Work out the finished part from the listing and answer in its coordinate system (mm). Face numbers are marked on the shaded views. A direction names the side the tool comes from. Coordinates: 2 decimals unless noted, no trailing zeros. Write item = value, one per line. Start each with the question number.
Q1. This flat-tipped pin is pushed along its axis until it touches: P1, Ø2, axis at y = 19.5, z = 2, coming from the -X side. Where does it stop, or does it pass through?
Q2. A tool of negligible diameter and unlimited length cuts with its end or side. For the marked faces 1 and 2, from which of +Z, -Z, +X, -X, +Y, -Y can it reach the whole face along a straight path? Write none if from no direction.
Q3. Straight lines are drawn through the part: line 1 along X through (y, z) = (29, 3); line 2 along X through (y, z) = (-27, 3.15); line 3 along Y through (x, z) = (-23.5, 3.65). For each, find the intervals that lie inside material, in ascending order.
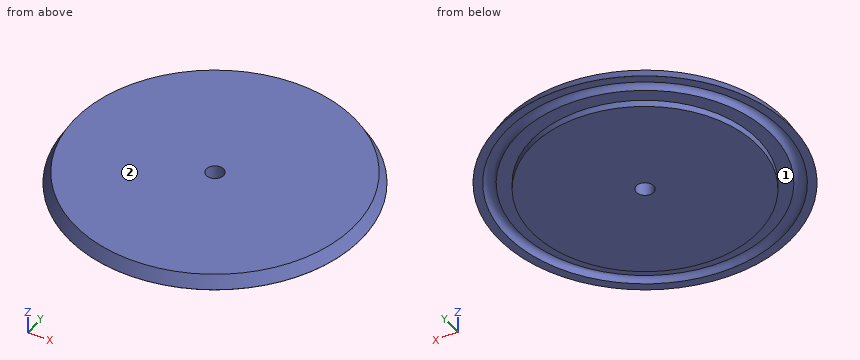
```python
from build123d import *

# Parameters (mm, degrees)
F2_R     = 2.6
F3_DEPTH = 5.501
F4_SIZE2 = 3.464102
F4_SIZE  = 2


with BuildPart() as f1:
    # F0 (on Front) → F1 (revolve)
    with BuildSketch(Plane.XZ):
        with BuildLine():
            Line((-34, 0), (0, 0))
            Line((0, 0), (0, 5.5))
            Line((0, 5.5), (-44, 5.5))
            Line((-44, 5.5), (-44, 2))
            Line((-44, 2), (-41.529162, 2))
            ThreePointArc((-41.529162, 2), (-39.8, 4.3), (-38.070838, 2))
            Line((-38.070838, 2), (-34, 2))
            Line((-34, 2), (-34, 0))
        make_face()
    revolve(axis=Axis((0, 0, 2.75), (0, 0, -1)))

    # F2 (on face) → F3 (cut, through all)
    with BuildSketch(Plane.XY.offset(5.5)):
        Circle(F2_R)
    extrude(amount=-F3_DEPTH, mode=Mode.SUBTRACT)

    # F4
    f4_edges = [f1.edges().sort_by_distance(p)[0] for p in [
        (44, 0, 5.5),
    ]]
    chamfer(f4_edges, length=F4_SIZE, length2=F4_SIZE2)


solid = f1.part
```
Findings below:
q1.P1 = -39.92
q2.face_1 = -Z
q2.face_2 = +Z, +X, -X, +Y, -Y
q3.line_1 = -32.35 to -29.73, -24.67 to 24.67, 29.73 to 32.35
q3.line_2 = -33.92 to -31.49, -26.91 to 26.91, 31.49 to 33.92
q3.line_3 = -36.09 to -33.82, -30.39 to 30.39, 33.82 to 36.09
